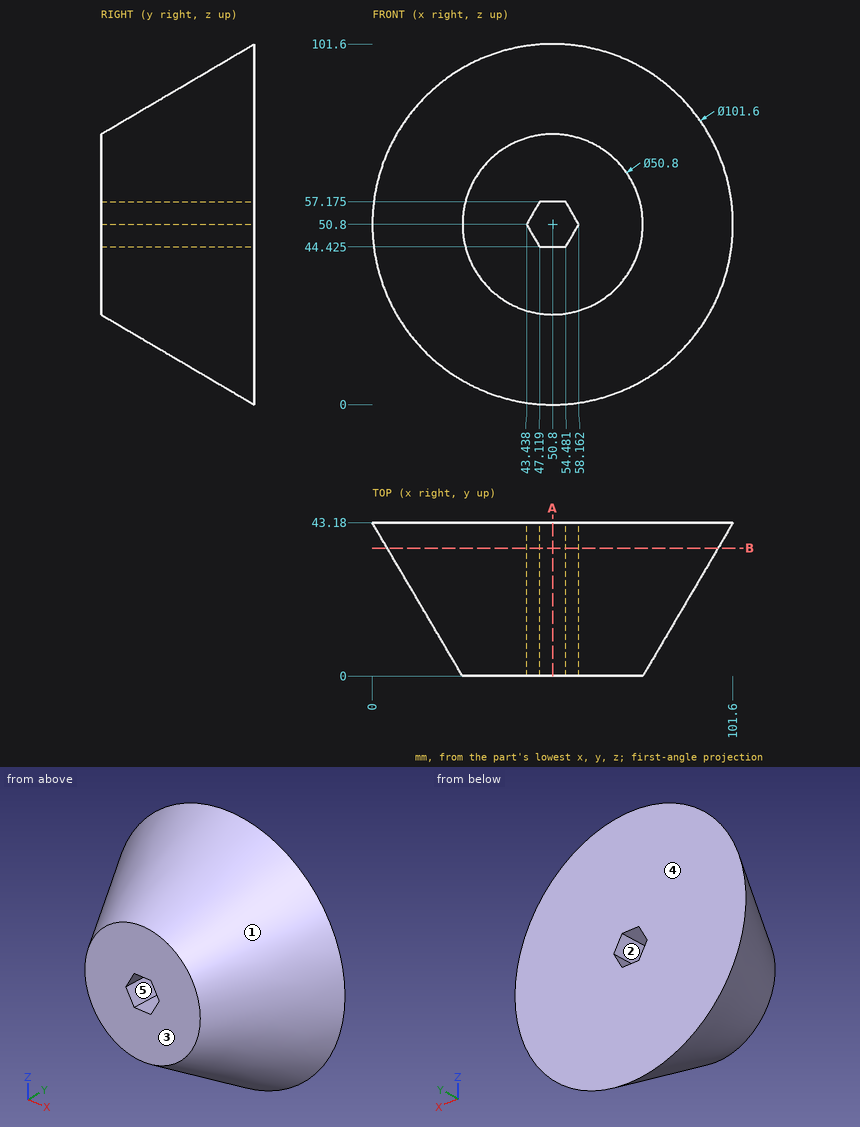
Geometry: see drawing. Coordinates: mm, zero at the bounding-box minimum. A direction names the side the tool comes from. Round coordinates to 2 decimals unless told otherwise and drop trailing zeros. Loops run counter-clockwise (first coordinate to the right, second up) from the corner with the lowest first, then second, coordinate; pieces in that order, holes last. Notation, with made-up numbers: (6.5, -29) - (14.5, -29) arc R25 ccw to (14.5, 4) - close; hole circle Ø8 at (47.25, 77). An arc over 180 degrees is marked (long way). One line per item, written item: value. Start each with the question number.
(1) Ray query, line 1 (X direction, y = 19.5, z = 53) (1 decimal); line 2 (Z direction, x = 54.5, y = 20.5) (1 decimal); line 3 (Z direction, x = 55.5, y = 14) (1 decimal). Return the intervals inside material, ascending. Write a range as [from, to].
(2) Section B-B, the plane y = 36. Return loops of the section in (x, z) (1 decimal), plus the area to 3 significant figures.
(3) Contact query for flat-ended pins moving along their axis: P1, Ø6, axis at x = 50, y = 13.5, coming from the +Z side; P2, Ø6, axis at x = 12.5, z = 60.5, coming from the -Y side (1 decimal); P3, Ø8, axis at x = 52.5, y = 23.5, coming from the -Z side. Output: stop coordinate, or through.
(4) Draft query along X for the marked faces 1, 2 and 3. Return one class per face: +X half, -X half, draft (parallel to the pull), parting line (faces both ways), or undercut.
(5) Access query for the marked faces 4 and 5. Directions: +Z, -Z, +X, -X, +Y, -Y. A direction counts if a zero-diameter tool reaches every point of the face in a straight line with its end or side. Return the directions, or none.
(6) Section A-A, the plane x = 50.8. Return loops of the section in (y, z) (1 decimal).
Results below:
1. line 1: [14, 44.7], [56.9, 87.6]
1. line 2: [13.5, 44.5], [57.1, 88.1]
1. line 3: [17.5, 46.2], [55.4, 84.1]
2. outline: circle Ø93.2 at (50.8, 50.8); hole (43.4, 50.8) - (47.1, 44.4) - (54.5, 44.4) - (58.2, 50.8) - (54.5, 57.2) - (47.1, 57.2) - close
2. area: 6,670 mm^2
3. P1: z = 85.9
3. P2: y = 18.9
3. P3: z = 9.25
4. face 1: parting line
4. face 2: undercut
4. face 3: draft
5. face 4: +Z, -Z, +X, -X, +Y
5. face 5: +Y, -Y
6. outline: (0, 25.4) - (43.2, 0) - (43.2, 44.4) - (0, 44.4) - close; (0, 57.2) - (43.2, 57.2) - (43.2, 101.6) - (0, 76.2) - close
